Here's how the part is built. I have some questions about the finished solid (model axes, mm). Face numbers are marked on the shaded views. A direction names the side the tool comes from. Round coordinates to 2 decimals unless told otherwise and drop trailing zeros. Order: outer loops, then holes, each group sorted by start corner. A loop starts at its lowest first (then second) coordinate and runs counter-clockwise, first axis right, second up. Notation, with made-up numbers: (5, 45.25) - (57, 45.25) arc R27 ccw to (57, 84.25) - close; hole circle Ø4 at (-25, -32.75). An arc over 180 degrees is marked (long way). One line per item, written item: value.
from build123d import *

# Parameters (mm, degrees)
F0_W     = 111.7562593253
F0_H     = 92.9139485481
F1_DEPTH = 45.974
F2_W     = 81.8422921002
F2_H     = 70.8807926811
F3_DEPTH = 109.728
F4_R     = 11.0212748346
F5_DEPTH = 176.022
F6_W     = 50.1861777157
F6_H     = 45.974
F7_DEPTH = 118.364


with BuildPart() as f1:
    # F0 (on Top) → F1 (new body, symmetric)
    with BuildSketch(Plane.XY):
        with Locations((-0.4647924884, 1.3352592527)):
            Rectangle(F0_W, F0_H)
    extrude(amount=F1_DEPTH, both=True)

    # F2 (on face) → F3 (cut, symmetric)
    with BuildSketch(Plane.XY.offset(45.974)):
        with Locations((-3.5118889064, 1.9688608032)):
            Rectangle(F2_W, F2_H)
    extrude(amount=F3_DEPTH, both=True, mode=Mode.SUBTRACT)

    # F4 (on face) → F5 (cut)
    with BuildSketch(Plane.YZ.offset(55.4133371742)):
        Circle(F4_R)
    extrude(amount=-F5_DEPTH, mode=Mode.SUBTRACT)

    # F6 (on face) → F7 (cut)
    with BuildSketch(Plane.XZ.offset(45.1217150214)):
        with Locations((1.5720045194, 22.987)):
            Rectangle(F6_W, F6_H)
    extrude(amount=-F7_DEPTH, mode=Mode.SUBTRACT)


solid = f1.part
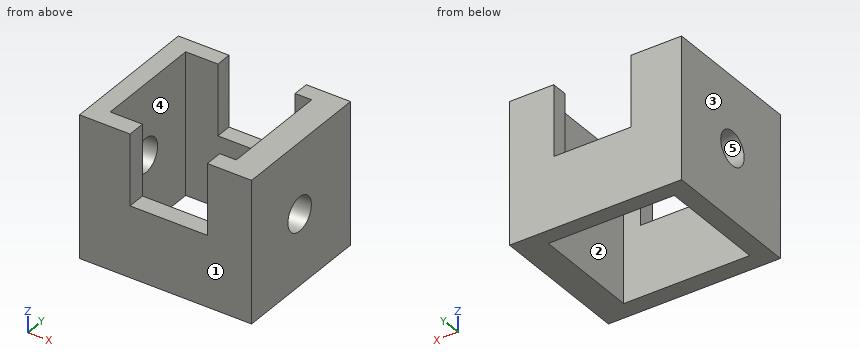
Q1. If we section it at D-D, the plane z = -19.5: Please give me the cut outline in (x, y), then the cut area to 3 significant figures.
Results list:
outline: (-56.34, -45.12) - (55.41, -45.12) - (55.41, 47.79) - (-56.34, 47.79) - close; hole (-44.43, -33.47) - (37.41, -33.47) - (37.41, 37.41) - (-44.43, 37.41) - close
area: 4,580 mm²
Q2. We'd pull the mould along X, two halves only. Please class the marked faces 3, 4 and 5: released by +X, released by -X, zero draft, split by the parting line, or undercut.
Results list:
face 3: released by -X
face 4: undercut
face 5: zero draft
Q3. If we section it at A-A, the plane z = 40.5: Please give me the cut outline in (x, y).
Results list:
outline: (-56.34, -45.12) - (-23.52, -45.12) - (-23.52, -33.47) - (-44.43, -33.47) - (-44.43, 37.41) - (-23.52, 37.41) - (-23.52, 47.79) - (-56.34, 47.79) - close; (26.67, -45.12) - (55.41, -45.12) - (55.41, 47.79) - (26.67, 47.79) - (26.67, 37.41) - (37.41, 37.41) - (37.41, -33.47) - (26.67, -33.47) - close
Q4. If we section it at C-C, the plane y = -20: Please give me the cut outline in (x, z), then the cut area to 3 significant figures.
Results list:
outline: (-56.34, -45.97) - (-44.43, -45.97) - (-44.43, 45.97) - (-56.34, 45.97) - close; (37.41, -45.97) - (55.41, -45.97) - (55.41, 45.97) - (37.41, 45.97) - close
area: 2,750 mm²
Q5. Which directions (+Z, -Z, +X, -X, +Y, -Y) give clear straight access to the entire face, cutting with the end or side of a thin tool? Please do the marked faces 1 and 2.
Results list:
face 1: +Z, -Z, +X, -X, -Y
face 2: +Z, -Z
Q6. If we section it at B-B, the plane x = 9.5: Please give me the cut outline in (y, z), then the cut area to 3 significant figures.
Results list:
outline: (-45.12, -45.97) - (-33.47, -45.97) - (-33.47, 0) - (-45.12, 0) - close; (37.41, -45.97) - (47.79, -45.97) - (47.79, 0) - (37.41, 0) - close
area: 1,010 mm²
Q7. Will this pin go through, and if not, where does the flat tip stop? pin 1 (11.5 mm diameter, centred on x = 1, y = 42, fed in from +Z).
Results list:
pin 1: z = 0
Q8. If I drill on line 1 along X through (y, z) = (9, -34); line 2 along Z through (x, y) = (49.5, 0); line 3 along Y through (x, z) = (27, 26), over which ranges is the centre line in solid material (lowest first)?
Results list:
line 1: -56.34 to -44.43, 37.41 to 55.41
line 2: -45.97 to -11.02, 11.02 to 45.97
line 3: -45.12 to -33.47, 37.41 to 47.79
